from build123d import *

# Parameters (mm, degrees)
SKETCH1_W           = 20
SKETCH1_H           = 10
BOSS_EXTRUDE1_DEPTH = 8
CUT_EXTRUDE2_DEPTH  = 8
SKETCH3_W           = 10
SKETCH3_H           = 3
BOSS_EXTRUDE2_DEPTH = 8
SKETCH4_R           = 1.25
CUT_EXTRUDE3_DEPTH  = 8
SKETCH5_R           = 1.25
CUT_EXTRUDE4_DEPTH  = 8


with BuildPart() as part:
    # Sketch1 → Boss-Extrude1 (new body)
    with BuildSketch(Plane.XY):
        with Locations((-58.400678179, 28.460872298)):
            Rectangle(SKETCH1_W, SKETCH1_H)
    extrude(amount=BOSS_EXTRUDE1_DEPTH)

    # Sketch2 → Cut-Extrude2 (cut)
    with BuildSketch(Plane.XY.offset(8)):
        with BuildLine():
            Line((-53.400678179, 33.460872298), (-53.400678179, 30.460872298))
            ThreePointArc((-53.400678179, 30.460872298), (-51.400678179, 28.460872298), (-53.400678179, 26.460872298))
            Line((-53.400678179, 26.460872298), (-68.400678179, 26.460872298))
            Line((-68.400678179, 26.460872298), (-68.400678179, 33.460872298))
            Line((-68.400678179, 33.460872298), (-53.400678179, 33.460872298))
        make_face()
    extrude(amount=-CUT_EXTRUDE2_DEPTH, mode=Mode.SUBTRACT)

    # Sketch3 → Boss-Extrude2 (add)
    with BuildSketch(Plane.XY.offset(8)):
        with Locations((-73.400678179, 24.960872298)):
            Rectangle(SKETCH3_W, SKETCH3_H)
    extrude(amount=-BOSS_EXTRUDE2_DEPTH)

    # Sketch4 → Cut-Extrude3 (cut)
    with BuildSketch(Plane(origin=(0, 26.460872298, 0), x_dir=(1, 0, 0), z_dir=(0, 1, 0))):
        with Locations(Location((-74.400678179, -4, 0), (0, 0, 270))):
            Circle(SKETCH4_R)
    extrude(amount=-CUT_EXTRUDE3_DEPTH, mode=Mode.SUBTRACT)

    # Sketch5 → Cut-Extrude4 (cut)
    with BuildSketch(Plane(origin=(0, 26.460872298, 0), x_dir=(1, 0, 0), z_dir=(0, 1, 0))):
        with Locations(Location((-64.400678179, -4, 0), (0, 0, 270))):
            Circle(SKETCH5_R)
    extrude(amount=-CUT_EXTRUDE4_DEPTH, mode=Mode.SUBTRACT)


solid = part.part
Model file for the job. Use its own axes, mm. A direction names the side the tool comes from. Round coordinates to 2 decimals unless told otherwise and drop trailing zeros. Loops run counter-clockwise (first coordinate to the right, second up) from the corner with the lowest first, then second, coordinate; pieces in that order, holes last. Notation, with made-up numbers: M -21.5,71.5 L 8.5,71.5 A28 cw 8.5,89.5 Z; hole C -1,26.5 d10. An arc over 180 degrees is marked long. One line per question, with ' | ' between items.
1) 3-axis set-ups, long thin cutter, end or side, ignore diameter. For faces 1 (the flat face through (-78.401, 25, 4)), 2 (the flat face through (-53.401, 32, 4)): which of +Z, -Z, +X, -X, +Y, -Y reach the whole face in a straight line?
Solved:
face 1: +Z, -Z, -X, +Y, -Y | face 2: +Z, -Z, -X, +Y
2) Band-saw the part on A-A (z = 4). Give the cut face in (x, y), then the cut area to 3 significant figures.
Solved:
outline: M -78.4,23.46 L -75.65,23.46 L -75.65,26.46 L -78.4,26.46 Z; M -73.15,23.46 L -65.65,23.46 L -65.65,26.46 L -73.15,26.46 Z; M -63.15,23.46 L -48.4,23.46 L -48.4,33.46 L -53.4,33.46 L -53.4,30.46 A2 cw -53.4,26.46 L -63.15,26.46 Z | area: 104 mm²
3) Mould opens along Y. For faces 3 (the flat face through (-64, 23.461, 6)), 4 (the cylindrical face through (-51.4, 28.5, 4.1)), 5 (the cylindrical face through (-65.51, 24.98, 4.58)), 6 (the flat face through (-66, 26.461, 4)) say: +Y half, -Y half, draft (parallel to the pull), parting line (faces both ways), or undercut.
Solved:
face 3: -Y half | face 4: undercut | face 5: draft | face 6: +Y half
4) Flat gauge pins, fed straight in: pin 1 (3 mm diameter, centred on x = -74.4, z = 4, fed in from -Y); pin 2 (2.5 mm diameter, centred on y = 31.5, z = 5.5, fed in from -X). Where does each tip first touch, or does it go through?
Solved:
pin 1: stops at y = 23.46 | pin 2: stops at x = -53.4
5) Band-saw the part on B-B (x = -75.25). Give the cut face in (y, z).
Solved:
outline: M 23.46,0 L 26.46,0 L 26.46,3.08 L 23.46,3.08 Z; M 23.46,4.92 L 26.46,4.92 L 26.46,8 L 23.46,8 Z
6) Band-saw the part on D-D (x = -67). Give the cut face in (y, z).
Solved:
outline: M 23.46,0 L 26.46,0 L 26.46,8 L 23.46,8 Z
7) Band-saw the part on C-C (z = 1). Give the cut face in (x, y).
Solved:
outline: M -78.4,23.46 L -48.4,23.46 L -48.4,33.46 L -53.4,33.46 L -53.4,30.46 A2 cw -53.4,26.46 L -78.4,26.46 Z
8) Drill centre lines: line 1 along X through (y, z) = (24.65, 4); line 2 along Y through (x, z) = (-59, 2.5); line 3 along X through (y, z) = (27.5, 6.75). Where is each one in solid material? Low to high.
Solved:
line 1: x = -78.4 to -75.65, -73.15 to -65.65, -63.15 to -48.4 | line 2: y = 23.46 to 26.46 | line 3: x = -51.65 to -48.4
